```python
from build123d import *

# Parameters (mm, degrees)
SKETCH1_W                 = 45.5
SKETCH1_H                 = 45
BOSS_EXTRUDE1_DEPTH       = 33
CUT_EXTRUDE1_DEPTH        = 46
CUT_EXTRUDE2_DEPTH        = 46
CUT_EXTRUDE4_DEPTH        = 46
M5X0_8_TAPPED_HOLE1_D     = 4.2
M5X0_8_TAPPED_HOLE1_DEPTH = 15.6
M5X0_8_TAPPED_HOLE1_TIP   = 1.2618073
CHAMFER1_SIZE             = 0.5


with BuildPart() as part:
    # Sketch1 → Boss-Extrude1 (new body)
    with BuildSketch(Plane(origin=(0, 0, -13.05), x_dir=(-1, 0, 0), z_dir=(0, 0, -1))):
        Rectangle(SKETCH1_W, SKETCH1_H)
    extrude(amount=-BOSS_EXTRUDE1_DEPTH)

    # Sketch2 → Cut-Extrude1 (cut, through all)
    with BuildSketch(Plane(origin=(0, 22.5, 0), x_dir=(-1, 0, 0), z_dir=(0, 1, 0))):
        Polygon((-21.2, -13.05), (-21.2, 9.45), (-22.75, 11.95), (-22.75, -13.05), align=None)
    cut_extrude1 = extrude(amount=-CUT_EXTRUDE1_DEPTH, mode=Mode.SUBTRACT)

    # Mirror1: Cut-Extrude1 across plane
    add(cut_extrude1.mirror(Plane(origin=(0, 0, 0), x_dir=(0, 0, 1), z_dir=(1, 0, 0))), mode=Mode.SUBTRACT)

    # Sketch3 → Cut-Extrude2 (cut, through all)
    with BuildSketch(Plane(origin=(0, 22.5, 0), x_dir=(-1, 0, 0), z_dir=(0, 1, 0))):
        Polygon((-10.5, 19.95), (-9.5, 18.95), (9.5, 18.95), (10.5, 19.95), align=None)
    extrude(amount=-CUT_EXTRUDE2_DEPTH, mode=Mode.SUBTRACT)

    # Sketch5 → Cut-Extrude4 (cut, through all)
    with BuildSketch(Plane(origin=(0, 22.5, 0), x_dir=(-1, 0, 0), z_dir=(0, 1, 0))):
        Polygon((-7.250013867, -13.05), (7.250013867, -13.05), (0, 2.768211411), align=None)
    extrude(amount=-CUT_EXTRUDE4_DEPTH, mode=Mode.SUBTRACT)

    # Sketch6 → Cut-Revolve1 (revolve, cut)
    with BuildSketch(Plane.XY.offset(-0.05)):
        Polygon((14, 22.5), (0, 22.5), (0, -22.5), (14, -22.5), (14, -19.8), (8, -19.8), (8, 19.8), (14, 19.8), align=None)
    revolve(axis=Axis((0, 22.5, -0.05), (0, -1, 0)), mode=Mode.SUBTRACT)

    # M5x0.8 Tapped Hole1
    with Locations(Plane.XY.offset(19.95)):
        with Locations((-16, -15), (16, 15), (16, -15), (-16, 15)):
            Hole(M5X0_8_TAPPED_HOLE1_D / 2, depth=M5X0_8_TAPPED_HOLE1_DEPTH)
            with Locations((0, 0, -(M5X0_8_TAPPED_HOLE1_DEPTH + M5X0_8_TAPPED_HOLE1_TIP / 2))):  # 118° drill point
                Cone(0, M5X0_8_TAPPED_HOLE1_D / 2, M5X0_8_TAPPED_HOLE1_TIP, mode=Mode.SUBTRACT)

    # Chamfer1
    chamfer1_edges = [part.edges().sort_by_distance(p)[0] for p in [
        (14.225006933, -22.5, -13.05),
        (16.625, -22.5, 19.95),
        (21.975, -22.5, 10.7),
        (21.2, -22.5, -1.8),
        (21.2, 22.5, -1.8),
        (21.975, 22.5, 10.7),
        (-14.225006933, 22.5, -13.05),
        (-21.2, 22.5, -1.8),
        (-21.975, 22.5, 10.7),
        (-21.2, -22.5, -1.8),
        (-21.975, -22.5, 10.7),
        (-16.625, -22.5, 19.95),
        (16.625, 22.5, 19.95),
        (-10, -22.5, 19.45),
        (0, -22.5, 18.95),
        (10, -22.5, 19.45),
        (10, 22.5, 19.45),
        (0, 22.5, 18.95),
        (-10, 22.5, 19.45),
        (-14.225006933, -22.5, -13.05),
        (14.225006933, 22.5, -13.05),
        (-7.065034848, -22.5, -12.646409431),
        (-7.065034848, 22.5, -12.646409431),
        (7.065034848, 22.5, -12.646409431),
        (7.065034848, -22.5, -12.646409431),
        (0, 22.5, 13.95),
        (0, -22.5, 13.95),
        (-22.75, -22.5, 15.95),
        (22.75, -22.5, 15.95),
        (22.75, 22.5, 15.95),
        (-22.75, 22.5, 15.95),
        (-16.625, 22.5, 19.95),
    ]]
    chamfer(chamfer1_edges, length=CHAMFER1_SIZE)


solid = part.part
```
The listing builds one solid part. Answer for the finished solid, in the listing's coordinates (mm). A direction names the side the tool comes from. Coordinates: 2 decimals unless noted, no trailing zeros. Loops run counter-clockwise (first coordinate to the right, second up) from the corner with the lowest first, then second, coordinate; pieces in that order, holes last. Notation, with made-up numbers: (-37.5, 37.25) -> (-15.5, 37.25) arc R16 ccw to (-15.5, 65.25) -> close; hole circle Ø10 at (-7.75, -25.75). An arc over 180 degrees is marked (long way). Return JSON: item names as keys, results as strings. Group by question number.
(1) Find the intervals of material crossed by probe 1 along Y at (x, z) = (16, 16.5); probe 2 along X at (y, z) = (-15, 14.5); probe 3 along X at (y, z) = (-3, -0.05), in increasing order. Write a range as from..to.
(2) Given pin 1 Ø8 at (y, z) = (-4.5, 4.5) entering from +X; pin 2 Ø4 at (x, z) = (7, -9.5) entering from +Y; pin 3 Ø5.5 at (x, y) = (4, -3) entering from +Z, each flat-ended and moving along its own axis, determine where each tip first touches the part or whether it passes through.
(3) Which of the six approach directions +Z, -Z, +X, -X, +Y, -Y give full straight-line access (tool end or side, diameter ignored) to faces 5 (the flat face through (0, -19.8, 10)), 6 (the flat face through (5.79, 0.31, -9.86)), 7 (the cylindrical face through (-17.13, 16.77, 12.04)), 8 (the flat face through (-10.11, -22.25, 19.21)), 9 (the flat face through (-21.2, 0, -2))?
(4) A cutting plane is placed at B-B on z = 11. Count the separate pieces of the cut face and the enclosed holes in it, and give its area (3 significant figures).
(5) A cutting plane is placed at A-A on y = 3. Write down the section's boundary in (x, z).
(6) Determine the mould class of faces 1 (the flat face through (21.2, 0, -2)), 2 (the flat face through (-5.83, 0.31, -9.95)), 3 (the flat face through (17, 0, 19.95)), 4 (the flat face through (-21.717, 22.246, 10.751)) for opening direction X: released by +X, released by -X, zero draft, split by the parting line, or undercut.
The answers:
{
 "1": {"probe 1": "y = -22.5..-17.1, -12.9..12.9, 17.1..22.5", "probe 2": "x = -22.75..-18.1, -13.9..13.9, 18.1..22.75", "probe 3": "x = -21.2..-8, 8..21.2"},
 "2": {"pin 1": "stops at x = 21.2", "pin 2": "stops at y = 19.8", "pin 3": "stops at z = 18.95"},
 "3": {"face 5": "-Y", "face 6": "-Z, +Y, -Y", "face 7": "+Z", "face 8": "+Z, -Y", "face 9": "-Z, -X, +Y, -Y"},
 "4": {"separate pieces": "1", "enclosed holes": "4", "area": "1,840 mm^2"},
 "5": {"outline": "(-22.75, 11.95) -> (-21.2, 9.45) -> (-21.2, -13.05) -> (-7.25, -13.05) -> (-4.36, -6.75) arc R8 cw (long way) to (4.36, -6.75) -> (7.25, -13.05) -> (21.2, -13.05) -> (21.2, 9.45) -> (22.75, 11.95) -> (22.75, 19.95) -> (10.5, 19.95) -> (9.5, 18.95) -> (-9.5, 18.95) -> (-10.5, 19.95) -> (-22.75, 19.95) -> close"},
 "6": {"face 1": "released by +X", "face 2": "undercut", "face 3": "zero draft", "face 4": "released by -X"}
}
